from build123d import *

# Parameters (mm, degrees)
SKETCH1_W           = 22.5
SKETCH1_H           = 22.7
BOSS_EXTRUDE1_DEPTH = 11.8
SKETCH2_W           = 4.7
SKETCH2_H           = 2.5
BOSS_EXTRUDE2_DEPTH = 11.8
SKETCH3_W           = 4.7
SKETCH3_H           = 2.5
BOSS_EXTRUDE3_DEPTH = 11.8
SKETCH4_R           = 5.9
BOSS_EXTRUDE4_DEPTH = 4
SKETCH5_R           = 2.9
BOSS_EXTRUDE5_DEPTH = 4
SKETCH6_R           = 1
SKETCH6_W           = 2.3
SKETCH6_H           = 1.3
CUT_EXTRUDE5_DEPTH  = 28.059240566
SKETCH8_R           = 1
SKETCH8_W           = 2.3
SKETCH8_H           = 1.3
CUT_EXTRUDE7_DEPTH  = 28.059240566
SKETCH9_R           = 2.3
SKETCH9_R_2         = 0.85
BOSS_EXTRUDE7_DEPTH = 3.2


with BuildPart() as part:
    # Sketch1 → Boss-Extrude1 (new body)
    with BuildSketch(Plane(origin=(0, 0, 0), x_dir=(1, 0, 0), z_dir=(0, 1, 0))):
        with Locations((0, -0.432106599)):
            Rectangle(SKETCH1_W, SKETCH1_H)
    extrude(amount=BOSS_EXTRUDE1_DEPTH)

    # Sketch2 → Boss-Extrude2 (add)
    with BuildSketch(Plane(origin=(0, 11.8, 0), x_dir=(1, 0, 0), z_dir=(0, 1, 0))):
        with Locations((13.6, 5.367893401)):
            Rectangle(SKETCH2_W, SKETCH2_H)
    extrude(amount=-BOSS_EXTRUDE2_DEPTH)

    # Sketch3 → Boss-Extrude3 (add)
    with BuildSketch(Plane(origin=(0, 11.8, 0), x_dir=(1, 0, 0), z_dir=(0, 1, 0))):
        with Locations((-13.6, 5.367893401)):
            Rectangle(SKETCH3_W, SKETCH3_H)
    extrude(amount=-BOSS_EXTRUDE3_DEPTH)

    # Sketch4 → Boss-Extrude4 (add)
    with BuildSketch(Plane(origin=(0, 0, -10.917893401), x_dir=(-1, 0, 0), z_dir=(0, 0, -1))):
        with Locations((5.35, 5.9)):
            Circle(SKETCH4_R)
    extrude(amount=BOSS_EXTRUDE4_DEPTH)

    # Sketch5 → Boss-Extrude5 (add)
    with BuildSketch(Plane(origin=(0, 0, -14.917893401), x_dir=(-1, 0, 0), z_dir=(0, 0, -1))):
        with Locations((-0.55, 5.9)):
            Circle(SKETCH5_R)
    extrude(amount=-BOSS_EXTRUDE5_DEPTH)

    # Sketch6 → Cut-Extrude5 (cut, through all)
    with BuildSketch(Plane(origin=(0, 0, -6.617893401), x_dir=(-1, 0, 0), z_dir=(0, 0, -1))):
        with Locations((-13.65, 5.9)):
            Circle(SKETCH6_R)
        with Locations((-14.8, 5.9)):
            Rectangle(SKETCH6_W, SKETCH6_H)
    extrude(amount=-CUT_EXTRUDE5_DEPTH, mode=Mode.SUBTRACT)

    # Sketch8 → Cut-Extrude7 (cut, through all)
    with BuildSketch(Plane(origin=(0, 0, -6.617893401), x_dir=(-1, 0, 0), z_dir=(0, 0, -1))):
        with Locations((13.65, 5.9)):
            Circle(SKETCH8_R)
        with Locations((14.8, 5.9)):
            Rectangle(SKETCH8_W, SKETCH8_H)
    extrude(amount=-CUT_EXTRUDE7_DEPTH, mode=Mode.SUBTRACT)

    # Sketch9 → Boss-Extrude7 (add)
    with BuildSketch(Plane(origin=(0, 0, -14.917893401), x_dir=(-1, 0, 0), z_dir=(0, 0, -1))):
        with Locations((5.35, 5.842855954)):
            Circle(SKETCH9_R)
        with Locations((5.35, 5.842855954)):
            Circle(SKETCH9_R_2, mode=Mode.SUBTRACT)
    extrude(amount=BOSS_EXTRUDE7_DEPTH)


solid = part.part
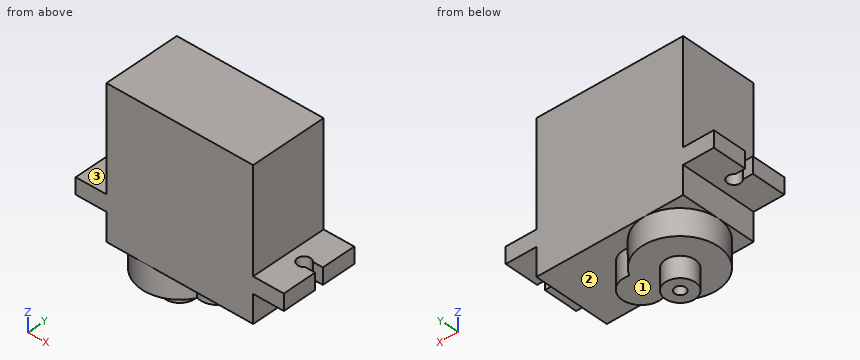
Build history of the part. All positions in model axes, mm. Face numbers are marked on the shaded views. A direction names the side the tool comes from. Round coordinates to 2 decimals unless told otherwise and drop trailing zeros. Loops run counter-clockwise (first coordinate to the right, second up) from the corner with the lowest first, then second, coordinate; pieces in that order, holes last. Notation, with made-up numbers: (-16, -40) -> (40, -40) arc R17 cw to (40, -23) -> close; hole circle Ø10 at (2, -18.75). An arc over 180 degrees is marked (long way). One line per item, written item: value. Start each with the question number.
Q1. Cut at A-A on x = -13.65. List the corners of the cut face in (y, z).
Q2. Cut at B-B on z = -5. List the corners of the cut face in (x, y).
Q3. Drop flat-ended pins along their axis: pin 1 Ø1.4 at (x, y) = (13, 4.5) entering from +Z; pin 2 Ø5 at (x, z) = (-3.5, -10.5) entering from -Y; pin 3 Ø5 at (y, z) = (4, 1) entering from +X; pin 4 Ø3.5 at (y, z) = (4, -8.5) entering from -X. Give the stop position or say it passes through.
Q4. 3-axis set-ups, long thin cutter, end or side, ignore diameter. For the marked faces 1, 2 and 3: which of +Z, -Z, +X, -X, +Y, -Y reach the whole face in a straight line?
Q5. Cut at D-D on y = 10.75. List the corners of the cut face in (x, z), plus the area to 3 significant figures.
Q6. Cut at C-C on x = 0.55. List the corners of the cut face in (y, z).
Q7. Probe line 1 along Y through (x, z) = (-13.65, -5.3); line 2 along Y through (x, z) = (-5.35, -16.7); line 3 along Z through (x, y) = (-11, 11). List the from-to ranges inside material, lowest first.
Computed:
1. outline: (0, -6.62) -> (4.9, -6.62) -> (4.9, -4.12) -> (0, -4.12) -> close; (6.9, -6.62) -> (11.8, -6.62) -> (11.8, -4.12) -> (6.9, -4.12) -> close
2. outline: (-15.95, 0) -> (15.95, 0) -> (15.95, 5.25) -> (14.41, 5.25) arc R1 cw (long way) to (14.41, 6.55) -> (15.95, 6.55) -> (15.95, 11.8) -> (-15.95, 11.8) -> (-15.95, 6.55) -> (-14.41, 6.55) arc R1 cw (long way) to (-14.41, 5.25) -> (-15.95, 5.25) -> close
3. pin 1: z = -4.12
3. pin 2: y = 0
3. pin 3: x = 11.25
3. pin 4: x = -11.25
4. face 1: -Z
4. face 2: -Z, +X
4. face 3: +Z, -X, +Y, -Y
5. outline: (-15.95, -6.62) -> (-11.25, -6.62) -> (-11.25, -10.92) -> (-8.71, -10.92) -> (-8.71, -14.92) -> (-1.99, -14.92) -> (-1.99, -10.92) -> (11.25, -10.92) -> (11.25, -6.62) -> (15.95, -6.62) -> (15.95, -4.12) -> (11.25, -4.12) -> (11.25, 11.78) -> (-11.25, 11.78) -> (-11.25, -4.12) -> (-15.95, -4.12) -> close
5. area: 561 mm²
6. outline: (0, -10.92) -> (3, -10.92) -> (3, -14.92) -> (8.8, -14.92) -> (8.8, -10.92) -> (11.8, -10.92) -> (11.8, 11.78) -> (0, 11.78) -> close
7. line 1: 0 to 4.9, 6.9 to 11.8
7. line 2: 3.54 to 4.99, 6.69 to 8.14
7. line 3: -10.92 to 11.78
